For this review, take the finished solid that the model builds, in its own axes (mm). A direction names the side the tool comes from. Coordinates: 2 decimals unless noted, no trailing zeros. Order: outer loops, then holes, each group sorted by start corner. A loop starts at its lowest first (then second) coordinate and runs counter-clockwise, first axis right, second up. Notation, with made-up numbers: (-14.75, 81.25) -> (43.25, 81.25) arc R15 ccw to (43.25, 91.25) -> close; hole circle Ø10 at (2.25, 9). An arc over 180 degrees is marked (long way). Return JSON: item names as keys, results as strings. Group by question number.
Item 1: Machinability: for faces 1 (the flat face through (12.7, 50, 6)), 2 (the conical face through (99.62, 23.11, 69.94)), 3 (the flat face through (103, 75.489, 71)), 4 (the flat face through (12.7, 32.6, 38.1)), 5 (the cylindrical face through (96.577, 68.287, 18.961)), which of the approach directions +Z, -Z, +X, -X, +Y, -Y give a long, thin tool a straight path to every point of the face, cutting with its end or side? Answer none if there is none.
Item 2: Take a section at B-B (z = 50). Count the separate pieces of the cut face and the enclosed holes in it, then the cut area to 3 significant figures.
Item 3: Take a section at A-A (z = 20.5). Write out the cut boundary in (x, y) (3 decimals), then the cut area to 3 significant figures.
Item 4: For line 1 along X through (y, z) = (77, 69); line 2 along Z through (x, y) = (72.5, 61); line 3 along Y through (x, z) = (78, 49), list the stretches that pass through material, from the lowest coordinate up.
Item 5: Insertion check: pin 1 (1.3 mm diameter, centred on y = 39, z = 69, fed in from -X); pin 2 (6.5 mm diameter, centred on y = 62.5, z = 7, fed in from +X); pin 3 (1.5 mm diameter, centred on y = 29.5, z = 47.5, fed in from +X). Each pin has a flat end and moves straight along its axis. Give the tip position at first contact, or say it passes through.
Item 6: Draft analysis for pull direction Y (two halves, no side actions). For faces 6 (the flat face through (60, 19.025, 6)), 7 (the flat face through (6.477, 76, 71)), 8 (the conical face through (58.85, 68.97, 69.94)), state which applies: +Y half, -Y half, draft (parallel to the pull), parting line (faces both ways), or undercut.
```python
from build123d import *

# Parameters (mm, degrees)
F0_W      = 106.2482
F0_H      = 81.9404
F1_DEPTH  = 88.0618
F2_W      = 62.9158
F2_H      = 12.7
F3_DEPTH  = 93.5482
F4_W      = 69.0118
F4_H      = 34.5059
F5_DEPTH  = 6.35
F6_W      = 69.0118
F6_H      = 34.5059
F7_DEPTH  = 12.7
F8_R      = 13.2461
F9_DEPTH  = 69.0118
F10_R     = 13.2461
F11_DEPTH = 53.975
F12_R     = 19.05
F13_DEPTH = 12.7
F14_R     = 3.175
F15_DEPTH = 12.7
F16_R     = 24.1173
F17_DEPTH = 4.3688
F17_TAPER = -25
F18_R     = 20.6375
F19_DEPTH = 4.3688
F20_R     = 13.2461
F21_DEPTH = 25.4
F23_R     = 17.399
F24_DEPTH = 25.4
F22_R     = 24.1173
F22_R_2   = 13.2461
F25_DEPTH = 4.3688
F25_TAPER = -25
F26_R     = 20.6375
F27_DEPTH = 4.3688
F28_R     = 13.2461
F29_DEPTH = 4.3688


with BuildPart() as f1:
    # F0 (on Top) → F1 (new body)
    with BuildSketch(Plane.XY):
        with Locations((53.1241, 40.9702)):
            Rectangle(F0_W, F0_H)
    extrude(amount=F1_DEPTH)

    # F2 (on face) → F3 (cut)
    with BuildSketch(Plane.YZ.offset(106.2482)):
        with Locations((50.4825, 6.35)):
            Rectangle(F2_W, F2_H)
    extrude(amount=-F3_DEPTH, mode=Mode.SUBTRACT)

    # F4 (on face) → F5 (cut)
    with BuildSketch(Plane.YZ.offset(106.2482)):
        with Locations((40.9829, 70.80885)):
            Rectangle(F4_W, F4_H)
        with BuildLine():
            Line((75.4888, 53.5559), (6.477, 53.5559))
            ThreePointArc((6.477, 53.5559), (40.9829, 19.05), (75.4888, 53.5559))
        make_face()
    extrude(amount=-F5_DEPTH, mode=Mode.SUBTRACT)

    # F6 (on face) → F7 (cut)
    with BuildSketch(Plane(origin=(0, 81.9404, 0), x_dir=(-1, 0, 0), z_dir=(0, 1, 0))):
        with Locations((-40.9829, 70.80885)):
            Rectangle(F6_W, F6_H)
        with BuildLine():
            Line((-6.477, 53.5559), (-75.4888, 53.5559))
            ThreePointArc((-75.4888, 53.5559), (-40.9829, 19.05), (-6.477, 53.5559))
        make_face()
    extrude(amount=-F7_DEPTH, mode=Mode.SUBTRACT)

    # F8 (on face) → F9 (cut)
    with BuildSketch(Plane.YZ.offset(99.8982)):
        with Locations((40.9829, 53.5559)):
            Circle(F8_R)
    extrude(amount=-F9_DEPTH, mode=Mode.SUBTRACT)

    # F10 (on face) → F11 (cut)
    with BuildSketch(Plane(origin=(0, 69.2404, 0), x_dir=(-1, 0, 0), z_dir=(0, 1, 0))):
        with Locations((-40.9829, 53.5559)):
            Circle(F10_R)
    extrude(amount=-F11_DEPTH, mode=Mode.SUBTRACT)

    # F12 (on face) → F13 (cut)
    with BuildSketch(Plane(origin=(0, 0, 0), x_dir=(0, -1, 0), z_dir=(-1, 0, 0))):
        with Locations((-40.9702, 53.5432)):
            Circle(F12_R)
    extrude(amount=-F13_DEPTH, mode=Mode.SUBTRACT)

    # F14 (on face) → F15 (cut)
    with BuildSketch(Plane(origin=(0, 0, 12.7), x_dir=(1, 0, 0), z_dir=(0, 0, -1))):
        with Locations((93.5482, -69.2404)):
            Circle(F14_R)
    extrude(amount=-F15_DEPTH, mode=Mode.SUBTRACT)

    # F16 (on face) → F17 (cut)
    with BuildSketch(Plane.YZ.offset(99.8982)):
        with Locations((40.9829, 53.5559)):
            Circle(F16_R)
    extrude(amount=-F17_DEPTH, taper=F17_TAPER, mode=Mode.SUBTRACT)

    # F18 (on face) → F19 (join)
    with BuildSketch(Plane.YZ.offset(95.5294)):
        with Locations((40.9829, 53.5559)):
            Circle(F18_R)
    extrude(amount=F19_DEPTH)

    # F20 (on face) → F21 (cut)
    with BuildSketch(Plane.YZ.offset(99.8982)):
        with Locations((40.9829, 53.5559)):
            Circle(F20_R)
    extrude(amount=-F21_DEPTH, mode=Mode.SUBTRACT)

    # F23 (on face) → F24 (cut)
    with BuildSketch(Plane(origin=(12.7, 0, 0), x_dir=(0, -1, 0), z_dir=(-1, 0, 0))):
        with Locations((-40.9702, 53.5432)):
            Circle(F23_R)
    extrude(amount=-F24_DEPTH, mode=Mode.SUBTRACT)

    # F22 (on face) → F25 (cut)
    with BuildSketch(Plane(origin=(0, 69.2404, 0), x_dir=(-1, 0, 0), z_dir=(0, 1, 0))):
        with Locations((-40.9829, 53.5559)):
            Circle(F22_R)
        with Locations((-40.9829, 53.5559)):
            Circle(F22_R_2, mode=Mode.SUBTRACT)
        with Locations((-40.9829, 53.5559)):
            Circle(F22_R)
    extrude(amount=-F25_DEPTH, taper=F25_TAPER, mode=Mode.SUBTRACT)

    # F26 (on face) → F27 (join)
    with BuildSketch(Plane(origin=(0, 64.8716, 0), x_dir=(-1, 0, 0), z_dir=(0, 1, 0))):
        with Locations((-40.9829, 53.5559)):
            Circle(F26_R)
    extrude(amount=F27_DEPTH)

    # F28 (on face) → F29 (cut, through all)
    with BuildSketch(Plane(origin=(0, 69.2404, 0), x_dir=(-1, 0, 0), z_dir=(0, 1, 0))):
        with Locations((-40.9829, 53.5559)):
            Circle(F28_R)
    extrude(amount=-F29_DEPTH, mode=Mode.SUBTRACT)


solid = f1.part
```
Findings below:
{
 "1": {"face 1": "-Z, +X, +Y", "face 2": "none", "face 3": "+Z, +X", "face 4": "-X", "face 5": "-Z"},
 "2": {"separate pieces": "3", "enclosed holes": "0", "area": "3,760 mm2"},
 "3": {"outline": "(0, 0) -> (106.248, 0) -> (106.248, 31.085) -> (99.898, 31.085) -> (99.898, 50.881) -> (106.248, 50.881) -> (106.248, 81.94) -> (50.881, 81.94) -> (50.881, 69.24) -> (31.085, 69.24) -> (31.085, 81.94) -> (0, 81.94) -> close; hole circle Ø6.35 at (93.548, 69.24)", "area": "8,300 mm2"},
 "4": {"line 1": "x = 0 to 6.48, 75.49 to 106.25", "line 2": "z = 12.7 to 88.06", "line 3": "y = 0 to 28.54, 53.42 to 81.94"},
 "5": {"pin 1": "stops at x = 38.1", "pin 2": "stops at x = 12.7", "pin 3": "stops at x = 99.9"},
 "6": {"face 6": "+Y half", "face 7": "draft", "face 8": "undercut"}
}
